from build123d import *

# Parameters (mm, degrees)
BOSS_EXTRU_1_DEPTH      = 3.175
CONG_1_R                = 6
CONG_2_R                = 2
ENL_V_MAT_EXTRU_2_DEPTH = 157.50531659973907
CONG_4_R                = 3
BOSS_EXTRU_2_DEPTH      = 3.175
CONG_5_R                = 2
CONG_6_R                = 3


with BuildPart() as part:
    # Esquisse1 → Boss.-Extru.1 (new body)
    with BuildSketch(Plane(origin=(0, 0, 0), x_dir=(0, 0, -1), z_dir=(1, 0, 0))):
        Polygon((-42.0728534805994, 0), (42.0728534805994, 0), (42.072853480599385, 84.94974746830529), (30.759144981614714, 96.26345596728963), (26.516504294495412, 92.02081528017037), (33.58757210636085, 84.94974746830486), (28.637824638054987, 79.99999999999906), (-42.07285348059938, 150.71067811865416), align=None)
    extrude(amount=BOSS_EXTRU_1_DEPTH)

    # Congé1
    cong_1_edges = [part.edges().sort_by_distance(p)[0] for p in [
        (1.5875, 84.94974746830529, -42.072853480599385),
    ]]
    fillet(cong_1_edges, radius=CONG_1_R)

    # Congé2
    cong_2_edges = [part.edges().sort_by_distance(p)[0] for p in [
        (1.5875, 92.02081528017037, -26.516504294495412),
        (1.5875, 96.26345596728963, -30.759144981614714),
    ]]
    fillet(cong_2_edges, radius=CONG_2_R)

    # Esquisse4 → Enlèv. mat.-Extru.2 (cut, through all)
    with BuildSketch(Plane(origin=(3.175, 0, 0), x_dir=(0, 0, -1), z_dir=(1, 0, 0))):
        Polygon((24.62411613906931, 72.7), (-34.07285348059938, 72.69999999999999), (-34.07285348059938, 131.39696961966868), align=None)
    extrude(amount=-ENL_V_MAT_EXTRU_2_DEPTH, mode=Mode.SUBTRACT)

    # Congé4
    cong_4_edges = [part.edges().sort_by_distance(p)[0] for p in [
        (1.5875, 150.71067811865416, 42.07285348059938),
        (1.5875, 131.39696961966868, 34.07285348059938),
        (1.5875, 72.7, -24.62411613906931),
        (1.5875, 72.69999999999999, 34.07285348059938),
    ]]
    fillet(cong_4_edges, radius=CONG_4_R)

    # Esquisse5 → Boss.-Extru.2 (add)
    with BuildSketch(Plane(origin=(3.175, 0, 0), x_dir=(0, 0, -1), z_dir=(1, 0, 0))):
        Polygon((30.759144981614842, 96.26345596728976), (26.51650429449542, 92.02081528017034), (0.7928932188133107, 117.74442635585244), (-4.15685424949237, 112.79467888754677), (28.637824638054987, 79.99999999999906), (37.8302127934801, 89.19238815542445), align=None)
    extrude(amount=-BOSS_EXTRU_2_DEPTH)

    # Congé5
    cong_5_edges = [part.edges().sort_by_distance(p)[0] for p in [
        (1.5875, 96.26345596728976, -30.759144981614842),
        (1.5875, 92.02081528017034, -26.51650429449542),
    ]]
    fillet(cong_5_edges, radius=CONG_5_R)

    # Congé6
    cong_6_edges = [part.edges().sort_by_distance(p)[0] for p in [
        (1.5875, 112.79467888754677, 4.15685424949237),
        (1.5875, 117.74442635585244, -0.7928932188133107),
    ]]
    fillet(cong_6_edges, radius=CONG_6_R)


solid = part.part
Model file for the job. Use its own axes, mm. A direction names the side the tool comes from. Coordinates: 2 decimals unless noted, no trailing zeros. Order: outer loops, then holes, each group sorted by start corner. A loop starts at its lowest first (then second) coordinate and runs counter-clockwise, first axis right, second up. Notation, with made-up numbers: M 47,13.5 L 57,13.5 A4 ccw 57,18.5 Z; hole C 17,82.25 d3. An arc over 180 degrees is marked long. Return JSON: item names as keys, results as strings.
1. Saw through at B-B (z = -1). Give the cut face in (x, y) (3 decimals), and give its area (3 significant figures).
Ans:
{"outline": "M 0,0 L 3.175,0 L 3.175,72.7 L 0,72.7 Z; M 0,96.324 L 3.175,96.324 L 3.175,116.495 L 0,116.495 Z", "area": "295 mm^2"}
2. Saw through at A-A (x = 2.1). Give the cut face in (y, z).
Ans:
{"outline": "M 0,-42.07 L 82.46,-42.07 A6 ccw 86.71,-40.32 L 94.85,-32.17 A2 ccw 94.85,-29.34 L 93.44,-27.93 A2 cw 93.44,-25.1 L 115.62,-2.91 A3 ccw 115.62,1.33 L 114.92,2.04 A3 cw 114.92,6.28 L 145.59,36.95 A3 ccw 143.47,42.07 L 0,42.07 Z; hole M 72.7,-17.38 A3 ccw 77.82,-19.5 L 126.28,28.95 A3 ccw 124.15,34.07 L 75.7,34.07 A3 ccw 72.7,31.07 Z"}
3. Pull direction Z, two halves, no side cores. Call faces 3 (the face through (3.175, 58, 1)), 4 (the face through (1.61, 90.72, -36.3)), 5 (the face through (2, 72.7, 7)), 6 (the face through (1.61, 102.388, 5.064)): +Z half, -Z half, draft (parallel to the pull), parting line (faces both ways), or undercut.
Ans:
{"face 3": "draft", "face 4": "-Z half", "face 5": "undercut", "face 6": "undercut"}
4. Drill centre lines: probe 1 along Y at (x, z) = (1.3, -20); probe 2 along Z at (x, y) = (2.1, 124.5); probe 3 along Z at (x, y) = (1.8, 120). Where is each one in solid material? Low to high.
Ans:
{"probe 1": "0 to 74.24, 77.16 to 98.54", "probe 2": "15.86 to 27.18, 34.05 to 42.07", "probe 3": "11.36 to 22.68, 34.07 to 42.07"}
5. Saw through at C-C (y = 97.5). Give the cut face in (x, z) (3 decimals), and give its area (3 significant figures).
Ans:
{"outline": "M 0,-21.037 L 3.175,-21.037 L 3.175,0.176 L 0,0.176 Z; M 0,34.073 L 3.175,34.073 L 3.175,42.073 L 0,42.073 Z", "area": "92.8 mm^2"}
6. Tool access for faces 1 (the face through (1.565, 114.038, 4.124)), 2 (the face through (1.565, 74.598, -20.172)): list every direction of +Z, -Z, +X, -X, +Y, -Y with a clear straight run to the whole face (end or side of a thin tool).
Ans:
{"face 1": "+X, -X, +Y", "face 2": "+X, -X"}
